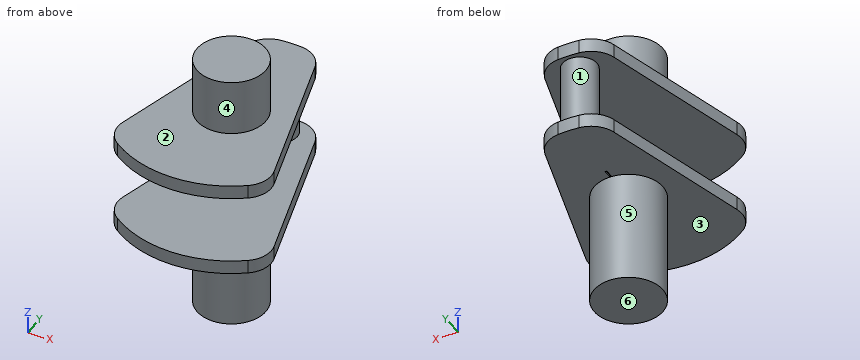
```python
from build123d import *

# Parameters (mm, degrees)
BOSS_EXTRUDE1_DEPTH = 0.8
SKETCH2_R           = 1
BOSS_EXTRUDE2_DEPTH = 2
SKETCH3_R           = 2
BOSS_EXTRUDE3_DEPTH = 3.26
SKETCH4_R           = 2
BOSS_EXTRUDE4_DEPTH = 3.34
SKETCH5_W           = 0.1
SKETCH5_H           = 0.5
CUT_EXTRUDE1_DEPTH  = 0.1


with BuildPart() as part:
    # Sketch1 → Boss-Extrude1 (new body)
    with BuildSketch(Plane.XY):
        with BuildLine():
            Line((-2.003843202, 5.298536735), (-4.412682198, -3.552198604))
            ThreePointArc((-4.412682198, -3.552198604), (-4.377352827, -4.505653519), (-3.805602751, -5.269476986))
            ThreePointArc((-3.805602751, -5.269476986), (0, -6.5), (3.805602751, -5.269476986))
            ThreePointArc((3.805602751, -5.269476986), (4.377352827, -4.505653519), (4.412682198, -3.552198604))
            Line((4.412682198, -3.552198604), (2.003843202, 5.298536735))
            ThreePointArc((2.003843202, 5.298536735), (1.490188902, 6.102578835), (0.610204082, 6.471294382))
            ThreePointArc((0.610204082, 6.471294382), (0, 6.5), (-0.610204082, 6.471294382))
            ThreePointArc((-0.610204082, 6.471294382), (-1.490188902, 6.102578835), (-2.003843202, 5.298536735))
        make_face()
    extrude(amount=BOSS_EXTRUDE1_DEPTH)

    # Sketch2 → Boss-Extrude2 (add)
    with BuildSketch(Plane.XY.offset(0.8)):
        with Locations((0, 5.26)):
            Circle(SKETCH2_R)
    extrude(amount=BOSS_EXTRUDE2_DEPTH)

    # Sketch3 → Boss-Extrude3 (add)
    with BuildSketch(Plane(origin=(0, 0, 0), x_dir=(-1, 0, 0), z_dir=(0, 0, -1))):
        Circle(SKETCH3_R)
    extrude(amount=BOSS_EXTRUDE3_DEPTH)

    # Mirror1: part across plane


with BuildPart() as part_1:
    add(part.part)
    add(part.part.mirror(Plane(origin=(0, 5.26, 2.8), x_dir=(1, 0, 0), z_dir=(0, 0, 1))))

    # Sketch4 → Boss-Extrude4 (add)
    with BuildSketch(Plane(origin=(0, 0, -3.26), x_dir=(-1, 0, 0), z_dir=(0, 0, -1))):
        Circle(SKETCH4_R)
    extrude(amount=BOSS_EXTRUDE4_DEPTH)

    # Sketch5 → Cut-Extrude1 (cut)
    with BuildSketch(Plane(origin=(0, 0, 0), x_dir=(-1, 0, 0), z_dir=(0, 0, -1))):
        with Locations((0.05, 2.269348072)):
            Rectangle(SKETCH5_W, SKETCH5_H)
    extrude(amount=-CUT_EXTRUDE1_DEPTH, mode=Mode.SUBTRACT)


solid = part_1.part
```
Source: CAD feature listing. Evaluate the final solid. Frame: model axes, mm. Face numbers are marked on the shaded views. A direction names the side the tool comes from. Round coordinates to 2 decimals unless told otherwise and drop trailing zeros. Loops run counter-clockwise (first coordinate to the right, second up) from the corner with the lowest first, then second, coordinate; pieces in that order, holes last. Notation, with made-up numbers: M 61,52 L 106,52 A17 cw 106,83 Z; hole C 2,9.25 d3. An arc over 180 degrees is marked long. Use a Markdown table: item, result. Add a question column.
1. Reachability of the marked faces 4, 5 and 6 from +Z, -Z, +X, -X, +Y, -Y: full face, straight path, thin tool, end or side. Return the list, or none.
2. Section query B-B on y = 1.75. Return the cut outline in (x, z), then the cut area to 3 significant figures.
3. Section query A-A on x = -1.25. Return the cut outline in (y, z), then the cut area to 3 significant figures.
4. Contact query for flat-ended pins moving along their axis: P1, Ø4, axis at x = -1.5, z = -1.5, coming from the -Y side; P2, Ø4, axis at x = 3.5, z = -2.5, coming from the +Y side; P3, Ø4, axis at x = 2.5, z = 1, coming from the +Y side. Output: stop coordinate, or through.
5. Section query D-D on x = -3.25. Return the cut outline in (y, z).
6. Line query: line 1 (Z direction, x = -2.25, y = 2.75); line 2 (Z direction, x = -1, y = -0.5); line 3 (Y direction, x = 0.75, z = -3.75). Output: solid intervals per line, ascending.
7. Mould query, pull axis Z, two halves, no side actions, for the marked faces 1, 2 and 3. Classes: pulls with the +Z half, pulls with the -Z half, needs draft (parallel to the pull), parting line crosses it, or undercut.
8. Section query C-C on z = 6. Return the cut outline in (x, y), then the cut area to 3 significant figures.
Reported:
| question | item | result |
|---|---|---|
| 1 | face 4 | +Z |
| 1 | face 5 | -Z |
| 1 | face 6 | -Z, +X, -X, +Y, -Y |
| 2 | outline | M -2.97,0 L -0.97,0 L -0.97,-6.6 L 0.97,-6.6 L 0.97,0 L 2.97,0 L 2.97,0.8 L -2.97,0.8 Z; M -2.97,4.8 L 2.97,4.8 L 2.97,5.6 L 0.97,5.6 L 0.97,8.86 L -0.97,8.86 L -0.97,5.6 L -2.97,5.6 Z |
| 2 | area | 28.6 mm² |
| 3 | outline | M -6.38,0 L -1.56,0 L -1.56,-6.6 L 1.56,-6.6 L 1.56,0 L 6.27,0 L 6.27,0.8 L -6.38,0.8 Z; M -6.38,4.8 L 6.27,4.8 L 6.27,5.6 L 1.56,5.6 L 1.56,8.86 L -1.56,8.86 L -1.56,5.6 L -6.38,5.6 Z |
| 3 | area | 51.0 mm² |
| 4 | P1 | stops at y = -6.5 |
| 4 | P2 | stops at y = 1.32 |
| 4 | P3 | stops at y = 6.48 |
| 5 | outline | M -5.63,0 L 0.72,0 L 0.72,0.8 L -5.63,0.8 Z; M -5.63,4.8 L 0.72,4.8 L 0.72,5.6 L -5.63,5.6 Z |
| 6 | line 1 | z = 0 to 0.8, 4.8 to 5.6 |
| 6 | line 2 | z = -6.6 to 0.8, 4.8 to 8.86 |
| 6 | line 3 | y = -1.85 to 1.85 |
| 7 | face 1 | undercut |
| 7 | face 2 | pulls with the +Z half |
| 7 | face 3 | pulls with the -Z half |
| 8 | outline | C 0,0 d4 |
| 8 | area | 12.6 mm² |
